Design review of the part shown in the three views and the two pictorial views. Dimensions are in mm from the part's minimum x, y and z. Round coordinates to 2 decimals unless told otherwise and drop trailing zeros. Loops run counter-clockwise (first coordinate to the right, second up) from the corner with the lowest first, then second, coordinate; pieces in that order, holes last. Notation, with made-up numbers: M 29,10.25 L 69,10.25 A11 ccw 69,15.25 Z; hole C -40,6 d2. An arc over 180 degrees is marked long. Return JSON: item names as keys, results as strings. Group by question number.
Q1. Draft analysis for pull direction Y (two halves, no side actions). For the marked faces 1 and 2, state which applies: pulls with the +Y half, pulls with the -Y half, needs draft (parallel to the pull), parting line crosses it, or undercut.
Q2. Consider section D-D (z = 199.5). State the section outline as (x, y) points, and give its area (3 significant figures).
Q3. Clearance check with flat-ended pins moving along their axes: pin 1 Ø12 at (x, y) = (14, 16) entering from +Z; pin 2 Ø6 at (y, z) = (12, 178) entering from -X; pin 3 Ø12 at (x, z) = (5, 114) entering from +Y; pin 4 Ø15 at (x, y) = (18.5, 23) entering from -Z. State where each tip first meets the part, or that it passes through.
Q4. Consider section A-A (x = 19). State the section outline as (y, z) points, and give its area (3 significant figures).
Q5. Consider section C-C (z = 174). State the section outline as (x, y) points.
Q6. To check wall thickness, follow line 1 along Y through (x, z) = (19, 205); line 2 along Y through (x, z) = (20, 29); line 3 along Z through (x, y) = (30.5, 6). State the ranges of each line that lie inside material, in increasing order.
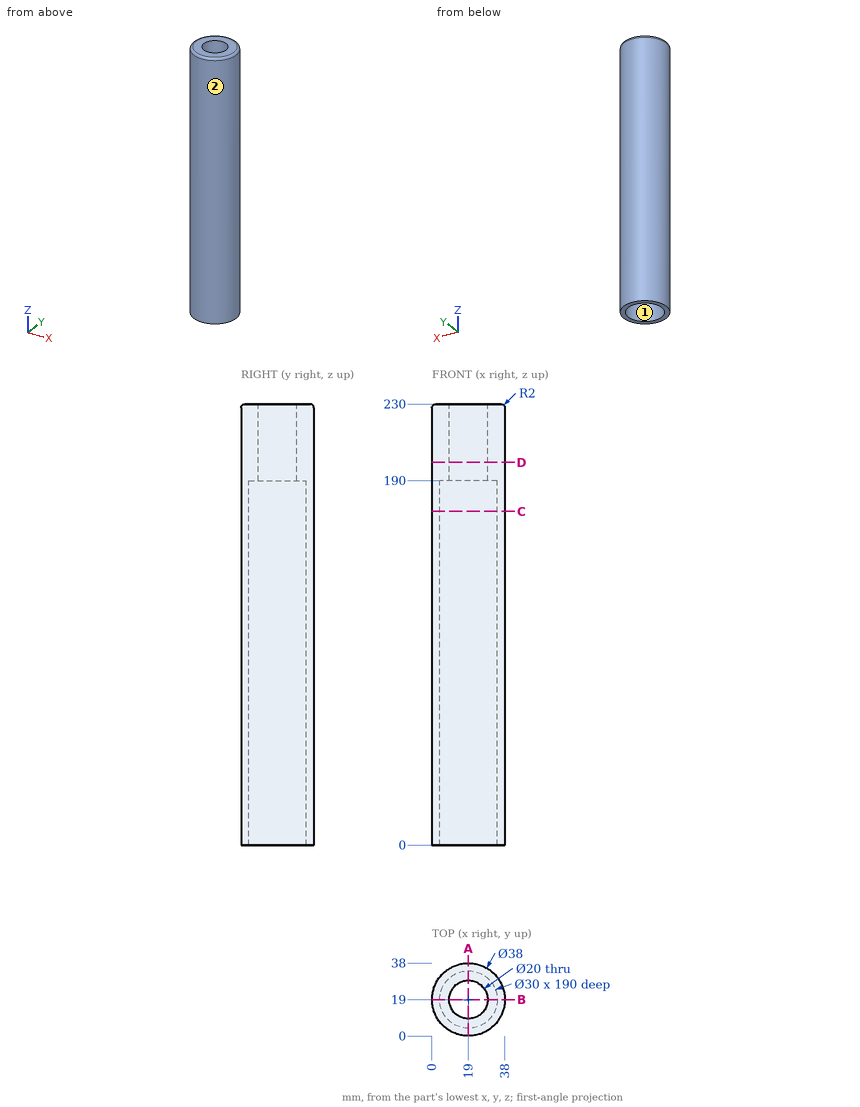
Values:
{
 "1": {"face 1": "undercut", "face 2": "parting line crosses it"},
 "2": {"outline": "C 19,19 d38; hole C 19,19 d20", "area": "820 mm2"},
 "3": {"pin 1": "stops at z = 230", "pin 2": "stops at x = 0.43", "pin 3": "stops at y = 36.23", "pin 4": "stops at z = 190"},
 "4": {"outline": "M 0,0 L 4,0 L 4,190 L 9,190 L 9,230 L 2,230 A2 ccw 0,228 Z; M 29,190 L 34,190 L 34,0 L 38,0 L 38,228 A2 ccw 36,230 L 29,230 Z", "area": "2,240 mm2"},
 "5": {"outline": "C 19,19 d38; hole C 19,19 d30"},
 "6": {"line 1": "y = 0 to 9, 29 to 38", "line 2": "y = 0.03 to 4.03, 33.97 to 37.97", "line 3": "z = 0 to 229.97"}
}
